Here's how the part is built. I have some questions about the finished solid (model axes, mm). Face numbers are marked on the shaded views. A direction names the side the tool comes from. Coordinates: 2 decimals unless noted, no trailing zeros. Write each loop counter-clockwise with the first axis right and the second up, starting at its lowest first coordinate (ties: lowest second). Pieces come first, ordered by that corner, then holes. Notation, with made-up numbers: (65, -25.5) -> (78, -25.5) arc R12 ccw to (78, -6.5) -> close; hole circle Ø6 at (27, 43.5). An arc over 180 degrees is marked (long way). Use a Markdown table: item, result. Add a question column.
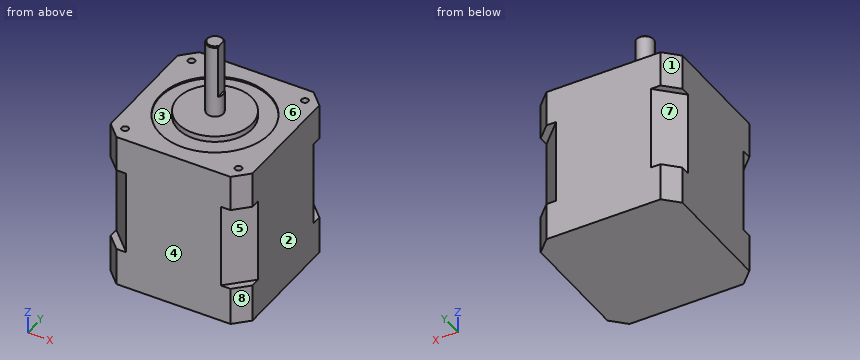
```python
from build123d import *

# Parameters (mm, degrees)
BOSS_EXTRU_1_DEPTH      = 11.2
BOSS_EXTRU_2_DEPTH      = 25.1
BOSS_EXTRU_3_DEPTH      = 10.6
ESQUISSE4_R             = 16.25
ENL_V_MAT_EXTRU_1_DEPTH = 0.5
ESQUISSE5_R             = 11
BOSS_EXTRU_4_DEPTH      = 1.7
ESQUISSE6_R             = 2.5
BOSS_EXTRU_5_DEPTH      = 22.2
CHANFREIN1_SIZE         = 0.3
ENL_V_MAT_EXTRU_2_DEPTH = 16
ESQUISSE8_R             = 1
ENL_V_MAT_EXTRU_3_DEPTH = 10


with BuildPart() as part:
    # Esquisse1 → Boss.-Extru.1 (new body)
    with BuildSketch(Plane.XY):
        Polygon((21, -16.9), (21, 16.9), (16.9, 21), (-16.9, 21), (-21, 16.9), (-21, -16.9), (-16.9, -21), (16.9, -21), align=None)
    extrude(amount=BOSS_EXTRU_1_DEPTH)

    # Esquisse2 → Boss.-Extru.2 (add)
    with BuildSketch(Plane.XY.offset(11.2)):
        Polygon((14, 21), (21, 14), (21, -14), (14, -21), (-14, -21), (-21, -14), (-21, 14), (-14, 21), align=None)
    extrude(amount=BOSS_EXTRU_2_DEPTH)

    # Esquisse3 → Boss.-Extru.3 (add)
    with BuildSketch(Plane.XY.offset(36.3)):
        Polygon((16.9, 21), (21, 16.9), (21, -16.9), (16.9, -21), (-16.9, -21), (-21, -16.9), (-21, 16.9), (-16.9, 21), align=None)
    extrude(amount=BOSS_EXTRU_3_DEPTH)

    # Esquisse4 → Enlèv. mat.-Extru.1 (cut)
    with BuildSketch(Plane.XY.offset(46.9)):
        Circle(ESQUISSE4_R)
    extrude(amount=-ENL_V_MAT_EXTRU_1_DEPTH, mode=Mode.SUBTRACT)

    # Esquisse5 → Boss.-Extru.4 (add)
    with BuildSketch(Plane.XY.offset(46.4)):
        Circle(ESQUISSE5_R)
    extrude(amount=BOSS_EXTRU_4_DEPTH)

    # Esquisse6 → Boss.-Extru.5 (add)
    with BuildSketch(Plane.XY.offset(48.1)):
        Circle(ESQUISSE6_R)
    extrude(amount=BOSS_EXTRU_5_DEPTH)

    # Chanfrein1
    chanfrein1_edges = [part.edges().sort_by_distance(p)[0] for p in [
        (-2.5, 0, 70.3),
    ]]
    chamfer(chanfrein1_edges, length=CHANFREIN1_SIZE)

    # Esquisse7 → Enlèv. mat.-Extru.2 (cut)
    with BuildSketch(Plane.XY.offset(70.3)):
        with BuildLine():
            Line((1.878163997, 1.65), (1.878163997, -1.65))
            ThreePointArc((1.878163997, -1.65), (2.5, 0), (1.878163997, 1.65))
        make_face()
    extrude(amount=-ENL_V_MAT_EXTRU_2_DEPTH, mode=Mode.SUBTRACT)

    # Esquisse8 → Enlèv. mat.-Extru.3 (cut)
    with BuildSketch(Plane.XY.offset(46.9)):
        with Locations((-16.8, 16.8)):
            Circle(ESQUISSE8_R)
        with Locations((-16.8, -16.8)):
            Circle(ESQUISSE8_R)
        with Locations((16.8, -16.8)):
            Circle(ESQUISSE8_R)
        with Locations((16.8, 16.8)):
            Circle(ESQUISSE8_R)
    extrude(amount=-ENL_V_MAT_EXTRU_3_DEPTH, mode=Mode.SUBTRACT)


solid = part.part
```
Q1. Suppose I cut it at C-C, the plane y = 12. Write out the boundary of the cut face in (x, z).
Q2. Please list where these lines run through material, in increasing order: line 1 (Y direction, x = 16.8, z = 39.75); line 2 (Y direction, x = 0, z = 46.5); line 3 (Z direction, x = -19, y = -8.5).
Q3. Thinking about a two-plate mould opening in X: for the marked faces 1, 2, 3 and 4, which applies, released by +X, released by -X, zero draft, split by the parting line, or undercut?
Q4. Suppose I cut it at A-A, the plane x = 0. Write out the boundary of the cut face in (y, z).
Q5. Will these pins go through, and if not, where does the flat tip stop? pin 1 (2.5 mm diameter, centred on x = 16.8, y = -16.8, fed in from -Z); pin 2 (2 mm diameter, centred on x = 17, y = 16.5, fed in from +Z); pin 3 (4 mm diameter, centred on y = -16.5, z = 32, fed in from +X); pin 4 (1.7 mm diameter, centred on y = 0.5, z = 59.5, fed in from +X).
Q6. Which directions (+Z, -Z, +X, -X, +Y, -Y) give clear straight access to the entire face, cutting with the end or side of a thin tool? Please do the marked faces 5, 6, 7 and 8.
Q7. Suppose I cut it at D-D, the plane z = 50. Write out the boundary of the cut face in (x, y).
Q8. Suppose I cut it at B-B, the plane z = 29.5. Write out the boundary of the cut face in (x, y).
Answer key:
| question | item | result |
|---|---|---|
| 1 | outline | (-21, 0) -> (21, 0) -> (21, 46.9) -> (10.96, 46.9) -> (10.96, 46.4) -> (-10.96, 46.4) -> (-10.96, 46.9) -> (-21, 46.9) -> close |
| 2 | line 1 | y = -21 to -17.8, -15.8 to 15.8, 17.8 to 21 |
| 2 | line 2 | y = -21 to -16.25, -11 to 11, 16.25 to 21 |
| 2 | line 3 | z = 0 to 46.9 |
| 3 | face 1 | released by -X |
| 3 | face 2 | released by +X |
| 3 | face 3 | undercut |
| 3 | face 4 | zero draft |
| 4 | outline | (-21, 0) -> (21, 0) -> (21, 46.9) -> (16.25, 46.9) -> (16.25, 46.4) -> (11, 46.4) -> (11, 48.1) -> (2.5, 48.1) -> (2.5, 70) -> (2.2, 70.3) -> (-2.2, 70.3) -> (-2.5, 70) -> (-2.5, 48.1) -> (-11, 48.1) -> (-11, 46.4) -> (-16.25, 46.4) -> (-16.25, 46.9) -> (-21, 46.9) -> close |
| 5 | pin 1 | stops at z = 0 |
| 5 | pin 2 | stops at z = 46.9 |
| 5 | pin 3 | stops at x = 20.5 |
| 5 | pin 4 | stops at x = 1.88 |
| 6 | face 5 | +X, -Y |
| 6 | face 6 | +Z |
| 6 | face 7 | -X, +Y |
| 6 | face 8 | +Z, -Z, +X, -Y |
| 7 | outline | circle Ø5 at (0, 0) |
| 8 | outline | (-21, -14) -> (-14, -21) -> (14, -21) -> (21, -14) -> (21, 14) -> (14, 21) -> (-14, 21) -> (-21, 14) -> close |
